Autodesk Inventor part; units mm, degrees
ref_plane "YZ Plane" through (0, 0, 0) normal (1, 0, 0) x (0, 1, 0)
ref_plane "XZ Plane" through (0, 0, 0) normal (0, 1, 0) x (-1, 0, 0)
ref_plane "XY Plane" through (0, 0, 0) normal (0, 0, 1) x (1, 0, 0)
sketch "Sketch1" plane through (0, 0, 0) normal (0, 0, 1) x (1, 0, 0)
  circle A0 centre (8.9, 0) radius 18.65
  circle A1 centre (23.4, 0) radius 1.65
  circle A2 centre (-5.6, 0) radius 1.65
  arc A3 (13.951, -13.4327) -> (21.5237, -6.826) centre (8.9, 0) ccw
  arc A4 (22.3604, -6.5571) -> (21.5237, -6.826) centre (22.0823, -7.128) ccw
  line L0 (22.3604, -6.5571) -> (23.5602, -7.1416)
  arc A5 (23.8417, -8.0126) -> (23.5602, -7.1416) centre (23.2821, -7.7125) ccw
  arc A6 (14.8123, -15.8902) -> (23.8417, -8.0126) centre (8.9, 0) ccw
  arc A7 (13.9876, -15.4932) -> (14.8123, -15.8902) centre (14.5909, -15.2951) ccw
  line L1 (13.9876, -15.4932) -> (13.5712, -14.2252)
  arc A8 (13.951, -13.4327) -> (13.5712, -14.2252) centre (14.1745, -14.0271) ccw
  line L2 (-4.5604, 6.5571) -> (-5.7602, 7.1416)
  arc A9 (-6.0417, 8.0126) -> (-5.7602, 7.1416) centre (-5.4821, 7.7125) ccw
  arc A10 (2.9877, 15.8902) -> (-6.0417, 8.0126) centre (8.9, 0) ccw
  arc A11 (3.8124, 15.4932) -> (2.9877, 15.8902) centre (3.2091, 15.2951) ccw
  line L3 (3.8124, 15.4932) -> (4.2288, 14.2252)
  arc A12 (3.849, 13.4327) -> (4.2288, 14.2252) centre (3.6255, 14.0271) ccw
  arc A13 (3.849, 13.4327) -> (-3.7237, 6.826) centre (8.9, 0) ccw
  arc A14 (-4.5604, 6.5571) -> (-3.7237, 6.826) centre (-4.2823, 7.128) ccw
  circle A15 centre (8.9, 0) radius 8.75
  line L4 (22.3604, 6.5571) -> (23.5602, 7.1416)
  arc A16 (21.5237, 6.826) -> (22.3604, 6.5571) centre (22.0823, 7.128) ccw
  arc A17 (21.5237, 6.826) -> (13.951, 13.4327) centre (8.9, 0) ccw
  arc A18 (13.5712, 14.2252) -> (13.951, 13.4327) centre (14.1745, 14.0271) ccw
  line L5 (13.9876, 15.4932) -> (13.5712, 14.2252)
  arc A19 (14.8123, 15.8902) -> (13.9876, 15.4932) centre (14.5909, 15.2951) ccw
  arc A20 (23.8417, 8.0126) -> (14.8123, 15.8902) centre (8.9, 0) ccw
  arc A21 (23.5602, 7.1416) -> (23.8417, 8.0126) centre (23.2821, 7.7125) ccw
  line L6 (-4.5604, -6.5571) -> (-5.7602, -7.1416)
  arc A22 (-3.7237, -6.826) -> (-4.5604, -6.5571) centre (-4.2823, -7.128) ccw
  arc A23 (-3.7237, -6.826) -> (3.849, -13.4327) centre (8.9, 0) ccw
  arc A24 (4.2288, -14.2252) -> (3.849, -13.4327) centre (3.6255, -14.0271) ccw
  line L7 (3.8124, -15.4932) -> (4.2288, -14.2252)
  arc A25 (2.9877, -15.8902) -> (3.8124, -15.4932) centre (3.2091, -15.2951) ccw
  arc A26 (-6.0417, -8.0126) -> (2.9877, -15.8902) centre (8.9, 0) ccw
  arc A27 (-5.7602, -7.1416) -> (-6.0417, -8.0126) centre (-5.4821, -7.7125) ccw
  circle A28 centre (-5.6, 0) radius 1.65
  circle A29 centre (23.4, 0) radius 1.65
  circle A30 centre (8.9, 0) radius 9.75
  line L8 (8.9, 0) -> (8.9, -30.48)
  circle A31 centre (8.9, -30.48) radius 2
  circle A32 centre (8.9, -30.48) radius 3.6
  line L9 (5.374, -31.2064) -> (-0.6495, -1.9673)
  line L10 (12.426, -31.2064) -> (18.4495, -1.9673)
  circle A33 centre (35.2965, 15.24) radius 2
  circle A34 centre (35.2965, 15.24) radius 3.6
  line L11 (8.9, 0) -> (35.2965, 15.24)
  line L12 (34.1625, 18.6568) -> (5.829, 9.2537)
  line L13 (37.6885, 12.5496) -> (15.3784, -7.2864)
  circle A35 centre (-17.4965, 15.24) radius 2
  circle A36 centre (-17.4965, 15.24) radius 3.6
  line L14 (8.9, 0) -> (-17.4965, 15.24)
  line L15 (-19.8885, 12.5496) -> (2.4216, -7.2864)
  line L16 (-16.3625, 18.6568) -> (11.971, 9.2537)
  circle A37 centre (-5.6, 0) radius 2
  circle A38 centre (-5.6, 0) radius 3.6
  circle A39 centre (23.4, 0) radius 2
  circle A40 centre (23.4, 0) radius 3.6
  line L17 (0.0034, -5.1364) -> (-6.4857, -3.4893)
  line L18 (-19.8885, 12.5496) -> (-8.4448, -2.2062)
  line L19 (37.6885, 12.5496) -> (26.2448, -2.2062)
  line L20 (17.7966, -5.1364) -> (24.2857, -3.4893)
  circle A41 centre (8.9, 0) radius 12.85
  point P0 (0, 0)
  point P1 (15.6508, -15.5526)
  point P2 (16.3247, -12.2811)
  point P3 (8.9, 10.2729)
  point P4 (1.4753, -12.2811)
  point P5 (2.1492, -15.5526)
  point P6 (13.7731, 11.8901)
  point P7 (4.0269, 11.8901)
  point P8 (16.7606, -10.1653)
  point P9 (21.001, -4.3231)
  point P10 (-3.201, -4.3231)
  point P11 (1.0394, -10.1653)
  dimension "d0" = 1
  dimension "d1" = 4
  dimension "d2" = 7.2
  dimension "d3" = 30.48
  dimension "d6" = 360
  dimension "d8" = 4
  dimension "d9" = 7.2
  dimension "d10" = 4
  dimension "d11" = 7.2
extrude "Extrusion1" add sketch "Sketch1" along normal blind 4 contours A0 L19 A40 L13 | A0 L13 L19 | L13 A40 A41 L11 A17 A16 L4 A21 A20 A0 | A0 L11 A34 L13 | L11 A20 L12 A0 | A0 L12 A34 L11 | A34 | A40 A41 L13 A39 | L13 A39 A41 A40 | L10 A32 L8 A0 | A0 L8 A41 L10 A3 A8 L1 A7 A6 | L11 A17 L12 A20 | A20 A21 L4 A16 A17 L11 | A41 A39 L13 A40 | A40 L13 L10 A30 L11 A41 | L8 A32 L9 A0 | A0 L9 A26 A25 L7 A24 A23 A41 L8 | A32 | A6 A7 L1 A8 A3 L10 | L20 A41 A40 | L16 A10 L14 A0 | A0 L14 A36 L16 | L11 A41 L12 A17 | A40 A41 L20 L13 | L13 A41 A40 | L11 A30 L16 L12 A41 | A41 L9 L15 A30 L8 | L8 A30 L13 L10 A41 | A41 L10 L20 | L14 A10 A9 L2 A14 A13 A41 A38 L15 A0 | A0 L15 A36 L14 | A36 | L16 A13 L14 A10 | L13 A41 A39 | L13 A30 L10 | L12 L16 A41 | L18 L15 A0 | A0 L15 A38 L18 | L9 A23 A24 L7 A25 A26 | A41 L17 L9 | L14 A13 A14 L2 A9 A10 | L16 A41 L14 A13 | A30 L12 L16 | L12 A30 L14 A41 L16 | A38 L15 A37 A41 | L15 L9 A30 | L15 A38 A41 L14 A30 L9 | L17 A41 A38 L15 | L17 A38 A41 | A38 A41 A37 L15 | A38 A41 L15 | L15 A41 A37 A38 | L15 A37 A41
fillet "Fillet1" radius 19.05 6 edges at (-3.201, -4.3231, 2) (1.0394, -10.1653, 2) (4.0269, 11.8901, 2) (13.7731, 11.8901, 2) (21.001, -4.3231, 2) (16.7606, -10.1653, 2)
sketch "Sketch2" plane through (0, 0, 4) normal (0, 0, 1) x (1, 0, 0)
  arc A0 (5.4731, -1.5453) -> (4.2552, -2.5573) centre (5.9714, -3.384) ccw
  arc A1 (4.2552, -2.5573) -> (4.6178, -3.1268) centre (8.9, 0) ccw
  arc A2 (4.6178, -3.1268) -> (6.05, -2.4513) centre (4.5948, -1.2219) ccw
  arc A3 (6.05, -2.4513) -> (6.7049, -3.0517) centre (8.9, 0) ccw
  arc A4 (6.7049, -3.0517) -> (6.1561, -4.5371) centre (8.0558, -4.3949) ccw
  arc A5 (6.1561, -4.5371) -> (6.7549, -4.849) centre (8.9, 0) ccw
  arc A6 (6.7549, -4.849) -> (7.6574, -3.5479) centre (5.7825, -3.2108) ccw
  arc A7 (7.6574, -3.5479) -> (8.5249, -3.7404) centre (8.9, 0) ccw
  arc A8 (8.5249, -3.7404) -> (8.7922, -5.3012) centre (10.3664, -4.2282) ccw
  arc A9 (8.7922, -5.3012) -> (9.4668, -5.2719) centre (8.9, 0) ccw
  arc A10 (9.4668, -5.2719) -> (9.5979, -3.6939) centre (7.8056, -4.3394) ccw
  arc A11 (9.5979, -3.6939) -> (10.4453, -3.4269) centre (8.9, 0) ccw
  arc A12 (10.4453, -3.4269) -> (11.4573, -4.6448) centre (12.284, -2.9286) ccw
  arc A13 (11.4573, -4.6448) -> (12.0268, -4.2822) centre (8.9, 0) ccw
  arc A14 (12.0268, -4.2822) -> (11.3513, -2.85) centre (10.1219, -4.3052) ccw
  arc A15 (11.3513, -2.85) -> (11.9517, -2.1951) centre (8.9, 0) ccw
  arc A16 (11.9517, -2.1951) -> (13.4371, -2.7439) centre (13.2949, -0.8442) ccw
  arc A17 (13.4371, -2.7439) -> (13.749, -2.1451) centre (8.9, 0) ccw
  arc A18 (13.749, -2.1451) -> (12.4479, -1.2426) centre (12.1108, -3.1175) ccw
  arc A19 (12.4479, -1.2426) -> (12.6404, -0.3751) centre (8.9, 0) ccw
  arc A20 (12.6404, -0.3751) -> (14.2012, -0.1078) centre (13.1282, 1.4664) ccw
  arc A21 (14.2012, -0.1078) -> (14.1719, 0.5668) centre (8.9, 0) ccw
  arc A22 (14.1719, 0.5668) -> (12.5939, 0.6979) centre (13.2394, -1.0944) ccw
  arc A23 (12.5939, 0.6979) -> (12.3269, 1.5453) centre (8.9, 0) ccw
  arc A24 (12.3269, 1.5453) -> (13.5448, 2.5573) centre (11.8286, 3.384) ccw
  arc A25 (13.5448, 2.5573) -> (13.1822, 3.1268) centre (8.9, 0) ccw
  arc A26 (13.1822, 3.1268) -> (11.75, 2.4513) centre (13.2052, 1.2219) ccw
  arc A27 (11.75, 2.4513) -> (11.0951, 3.0517) centre (8.9, 0) ccw
  arc A28 (11.0951, 3.0517) -> (11.6439, 4.5371) centre (9.7442, 4.3949) ccw
  arc A29 (11.6439, 4.5371) -> (11.0451, 4.849) centre (8.9, 0) ccw
  arc A30 (11.0451, 4.849) -> (10.1426, 3.5479) centre (12.0175, 3.2108) ccw
  arc A31 (10.1426, 3.5479) -> (9.2751, 3.7404) centre (8.9, 0) ccw
  arc A32 (9.2751, 3.7404) -> (9.0078, 5.3012) centre (7.4336, 4.2282) ccw
  arc A33 (9.0078, 5.3012) -> (8.3332, 5.2719) centre (8.9, 0) ccw
  arc A34 (8.3332, 5.2719) -> (8.2021, 3.6939) centre (9.9944, 4.3394) ccw
  arc A35 (8.2021, 3.6939) -> (7.3547, 3.4269) centre (8.9, 0) ccw
  arc A36 (7.3547, 3.4269) -> (6.3427, 4.6448) centre (5.516, 2.9286) ccw
  arc A37 (6.3427, 4.6448) -> (5.7732, 4.2822) centre (8.9, 0) ccw
  arc A38 (5.7732, 4.2822) -> (6.4487, 2.85) centre (7.6781, 4.3052) ccw
  arc A39 (6.4487, 2.85) -> (5.8483, 2.1951) centre (8.9, 0) ccw
  arc A40 (5.8483, 2.1951) -> (4.3629, 2.7439) centre (4.5051, 0.8442) ccw
  arc A41 (4.3629, 2.7439) -> (4.051, 2.1451) centre (8.9, 0) ccw
  arc A42 (4.051, 2.1451) -> (5.3521, 1.2426) centre (5.6892, 3.1175) ccw
  arc A43 (5.3521, 1.2426) -> (5.1596, 0.3751) centre (8.9, 0) ccw
  arc A44 (5.1596, 0.3751) -> (3.5988, 0.1078) centre (4.6718, -1.4664) ccw
  arc A45 (3.5988, 0.1078) -> (3.6281, -0.5668) centre (8.9, 0) ccw
  arc A46 (3.6281, -0.5668) -> (5.2061, -0.6979) centre (4.5606, 1.0944) ccw
  arc A47 (5.2061, -0.6979) -> (5.4731, -1.5453) centre (8.9, 0) ccw
  circle A48 centre (8.9, 0) radius 2.7343
  circle A49 centre (8.9, 27.5717) radius 23.8125
  circle A50 centre (8.9, 0) radius 3.7592
  line L0 (4.1375, 24.8221) -> (4.1375, 30.3213)
  line L1 (4.1375, 30.3213) -> (8.9, 33.071)
  line L2 (8.9, 33.071) -> (13.6625, 30.3213)
  line L3 (13.6625, 30.3213) -> (13.6625, 24.8221)
  line L4 (13.6625, 24.8221) -> (8.9, 22.0724)
  line L5 (8.9, 22.0724) -> (4.1375, 24.8221)
  line L6 (13.6625, 24.8221) -> (4.1375, 30.3213)
  line L7 (8.9, 33.071) -> (8.9, 22.0724)
  line L8 (4.1375, 24.8221) -> (13.6625, 30.3213)
  point P0 (0, 0)
  dimension "d15" = 47.625
  dimension "d16" = 9.525
  dimension "d17" = 9.525
  dimension "d18" = 9.525
properties part number "MotorHolder"
Model file for the job. Use its own axes, mm. A direction names the side the tool comes from. Round coordinates to 2 decimals unless told otherwise and drop trailing zeros. Loops run counter-clockwise (first coordinate to the right, second up) from the corner with the lowest first, then second, coordinate; pieces in that order, holes last. Notation, with made-up numbers: M -3.5,51 L 5.5,51 A22 ccw 5.5,88 Z; hole C 46.25,28 d11. An arc over 180 degrees is marked long. One line per question, with ' | ' between items.
1) 3-axis set-ups, long thin cutter, end or side, ignore diameter. For faces 5 (the flat face through (26.61, 16.15, 1.97)), 6 (the flat face through (9, 10, 0)): which of +Z, -Z, +X, -X, +Y, -Y reach the whole face in a straight line?
Solved:
face 5: +Z, -Z, +Y | face 6: -Z, +X, -X, +Y, -Y
2) Flat gauge pins, fed straight in: pin 1 (5 mm diameter, centred on x = 23.4, y = 0, fed in from -Z); pin 2 (3 mm diameter, centred on x = -17.5, y = 15.24, fed in from +Z); pin 3 (1 mm diameter, centred on x = -15, z = 1.5, fed in from -Y); pin 4 (1.5 mm diameter, centred on x = 17, z = 2, fed in from +Y). Where does each tip first touch, or does it go through?
Solved:
pin 1: stops at z = 0 | pin 2: passes through | pin 3: stops at y = 5.6 | pin 4: stops at y = 13.25
3) Band-saw the part on D-D (z = 1.05). Give the number of separate pieces and of enclosed holes in the cut face, then the cut area to 3 significant figures.
Solved:
separate pieces: 1 | enclosed holes: 6 | area: 944 mm²
4) Mould opens along Y. For faces 1 (the cylindrical face through (14.66, 12.69, 2.03)), 2 (the cylindrical face through (-7.598, -0.088, 1.972)), 3 (the flat face through (9, 10, 4)), 4 (the cylindrical face through (33.82, 13.89, 1.97)) say: +Y half, -Y half, draft (parallel to the pull), parting line (faces both ways), or undercut.
Solved:
face 1: +Y half | face 2: undercut | face 3: draft | face 4: undercut
5) Band-saw the part on B-B (y = -30.48). Give the cut face in (x, z).
Solved:
outline: M 5.22,0 L 6.9,0 L 6.9,4 L 5.22,4 Z; M 10.9,0 L 12.58,0 L 12.58,4 L 10.9,4 Z
6) Band-saw the part on A-A (x = 8.9). Give the cut face in (y, z), then the cut area to 3 significant figures.
Solved:
outline: M -34.08,0 L -32.48,0 L -32.48,4 L -34.08,4 Z; M -28.48,0 L -9.75,0 L -9.75,4 L -28.48,4 Z; M 9.75,0 L 12.85,0 L 12.85,4 L 9.75,4 Z | area: 93.7 mm²
7) Drill centre lines: line 1 along X through (y, z) = (0, 1.6); line 2 along Y through (x, z) = (10.5, 1.8); line 3 along X through (y, z) = (1.5, 1.15). Where is each one in solid material? Low to high.
Solved:
line 1: x = -10.16 to -7.6, -3.6 to -0.85, 18.65 to 21.4, 25.4 to 27.96 | line 2: y = -33.7 to -31.68, -29.28 to -9.62, 9.62 to 12.75 | line 3: x = -11.32 to -6.92, -4.28 to -0.73, 18.53 to 22.08, 24.72 to 29.12
8) Band-saw the part on C-C (y = 0). Give the cut face in (x, z), then the cut area to 3 significant figures.
Solved:
outline: M -10.16,0 L -7.6,0 L -7.6,4 L -10.16,4 Z; M -3.6,0 L -0.85,0 L -0.85,4 L -3.6,4 Z; M 18.65,0 L 21.4,0 L 21.4,4 L 18.65,4 Z; M 25.4,0 L 27.96,0 L 27.96,4 L 25.4,4 Z | area: 42.4 mm²
